Autodesk Inventor part; units mm, degrees
ref_plane "YZ Plane" through (0, 0, 0) normal (1, 0, 0) x (0, 1, 0)
ref_plane "XZ Plane" through (0, 0, 0) normal (0, 1, 0) x (-1, 0, 0)
ref_plane "XY Plane" through (0, 0, 0) normal (0, 0, 1) x (1, 0, 0)
sketch "草圖1" plane through (0, 0, 0) normal (0, 0, 1) x (1, 0, 0)
  line L0 (0, 0) -> (1.75, 0)
  line L1 (1.75, 0) -> (1.75, 60)
  line L2 (1.75, 60) -> (0, 60)
  line L3 (0, 60) -> (0, 0)
  dimension "d0" = 1.75
  dimension "d1" = 60
revolve "迴轉1" add sketch "草圖1" angle 360 about axis through (0, 60, 0) along (0, -1, 0)
sketch "草圖2" plane through (0, 0, 0) normal (0, 0, 1) x (1, 0, 0)
  line L0 (15, 0) -> (-15, 0)
  line L1 (-15, 0) -> (-15, 10)
  line L2 (-15, 10) -> (15, 10)
  line L3 (15, 10) -> (15, 0)
  point P0 (0, 0)
  dimension "d3" = 10
  dimension "d4" = 30
  dimension "d5" = 15
extrude "擠出1" add sketch "草圖2" along normal mid plane 10
chamfer "倒角1" distance 5 angle 45 2 edges at (-15, 10, 0) (15, 10, 0)
properties part number "車軸"
Source: CAD feature listing. Evaluate the final solid. Frame: model axes, mm. A direction names the side the tool comes from. Round coordinates to 2 decimals unless told otherwise and drop trailing zeros. Loops run counter-clockwise (first coordinate to the right, second up) from the corner with the lowest first, then second, coordinate; pieces in that order, holes last. Notation, with made-up numbers: M -36,5.25 L 4,5.25 A16 cw 4,33.25 Z; hole C 56,-5.5 d8. An arc over 180 degrees is marked long. Put each result on its own line as item: value.
(1) Ray query, line 1 (Y direction, x = -2, z = 4.75); line 2 (X direction, y = 9, z = -0.5); line 3 (Z direction, x = 1.5, y = 31). Return the intervals inside material, ascending. Write a range as [from, to].
Solutions:
line 1: [0, 10]
line 2: [-11, 11]
line 3: [-0.9, 0.9]
(2) Access query for faces 1 (the face through (1.617, 35.35, 0.67)), 2 (the face through (-15, 2, 0)). Directions: +Z, -Z, +X, -X, +Y, -Y. A direction counts if a zero-diameter tool reaches every point of the face in a straight line with its end or side. Return the directions, or none.
Solutions:
face 1: +Y
face 2: +Z, -Z, -X, +Y, -Y
(3) First-contact query: pin 1 (4 mm diameter, centred on y = 22, z = -3, fed in from -X); pin 2 (6 mm diameter, centred on y = 12, z = 4, fed in from -X); pin 3 (1 mm diameter, centred on y = 31.5, z = -2, fed in from -X). Flat tips, straight axial feed; report the tip coordinate or a pass-through.
Solutions:
pin 1: x = -1.44
pin 2: x = -11
pin 3: x = -0.9
(4) Section B-B, the plane z = 0. Return loops of the section in (x, y), and give its area (3 significant figures).
Solutions:
outline: M -15,0 L 15,0 L 15,5 L 10,10 L 1.75,10 L 1.75,60 L -1.75,60 L -1.75,10 L -10,10 L -15,5 Z
area: 450 mm²
(5) Section A-A, the plane x = 0. Return loops of the section in (y, z).
Solutions:
outline: M 0,-5 L 10,-5 L 10,-1.75 L 60,-1.75 L 60,1.75 L 10,1.75 L 10,5 L 0,5 Z
(6) Section D-D, the plane z = 4. Return loops of the section in (x, y).
Solutions:
outline: M -15,0 L 15,0 L 15,5 L 10,10 L -10,10 L -15,5 Z
(7) Section C-C, the plane y = 54.5. Return loops of the section in (x, z), and give its area (3 significant figures).
Solutions:
outline: C 0,0 d3.5
area: 9.62 mm²
